```python
from build123d import *

# Parameters (mm, degrees)
FILLET_1_R = 2


with BuildPart() as part:
    # Эскиз1 → Повернуть1 (revolve)
    with BuildSketch(Plane.XY, mode=Mode.PRIVATE) as revolve_1_sk:
        Polygon((0, 11.2), (20, 11.2), (20, 14.7), (16, 14.7), (16, 15), (2, 15), (2, 14.7), (0, 14.7), align=None)
    revolve(revolve_1_sk.sketch.rotate(Axis((0, 0, 0), (1, 0, 0)), 90), axis=Axis((0, 0, 0), (1, 0, 0)))

    # Скругление1
    fillet_1_edges = [part.edges().sort_by_distance(p)[0] for p in [
        (0, 0, -14.7),
    ]]
    fillet(fillet_1_edges, radius=FILLET_1_R - 0.0001)  # a hair under: the kernel refuses the full size


solid = part.part
```
Source: CAD feature listing. Evaluate the final solid. Frame: model axes, mm. A direction names the side the tool comes from. Round coordinates to 2 decimals unless told otherwise and drop trailing zeros. Order: outer loops, then holes, each group sorted by start corner. A loop starts at its lowest first (then second) coordinate and runs counter-clockwise, first axis right, second up. Notation, with made-up numbers: (-22, -7.75) -> (36, -7.75) arc R26 cw to (36, 14.25) -> close; hole circle Ø9 at (17.25, -18.5). An arc over 180 degrees is marked (long way). Use CSV: the item, a comma, the result in double quotes.
(1) First-contact query: pin 1 Ø1 at (x, y) = (4, -6) entering from +Z. Flat tip, straight axial feed; report the tip coordinate or a pass-through.
Report:
pin 1,"z = 13.96"
(2) Access query for faces 4 (the face through (0, 9, 7)), 5 (the face through (17.97, 14.35, -3.19)). Directions: +Z, -Z, +X, -X, +Y, -Y. A direction counts if a zero-diameter tool reaches every point of the face in a straight line with its end or side. Return the directions, or none.
Report:
face 4,"+Z, -Z, -X, +Y, -Y"
face 5,"+X"
(3) Ray query, L1, parallel to Y at x = 14.5, z = 0; L2, parallel to Y at x = 3.5, z = -7.5; L3, parallel to Z at x = 19.25, y = -3. Return the intervals inside material, ascending.
Report:
L1,"-15 to -11.2, 11.2 to 15"
L2,"-12.99 to -8.32, 8.32 to 12.99"
L3,"-14.39 to -10.79, 10.79 to 14.39"
(4) Pull-direction query (Z, two-part tool) for faces 1 (the face through (20, 11, 3)), 2 (the face through (8.9, -12.65, 8.06)), 3 (the face through (10.14, -0.49, -11.19)); classes: +Z half, -Z half, draft (parallel to the pull), parting line (faces both ways), or undercut.
Report:
face 1,"draft"
face 2,"parting line"
face 3,"undercut"
(5) Section C-C on x = 11.25. Return the cut outline in (y, z).
Report:
outline,"circle Ø30 at (0, 0); hole circle Ø22.4 at (0, 0)"
(6) Section D-D on x = 17.5. Return the cut outline in (y, z), and give its area (3 significant figures).
Report:
outline,"circle Ø29.4 at (0, 0); hole circle Ø22.4 at (0, 0)"
area,"285 mm^2"
